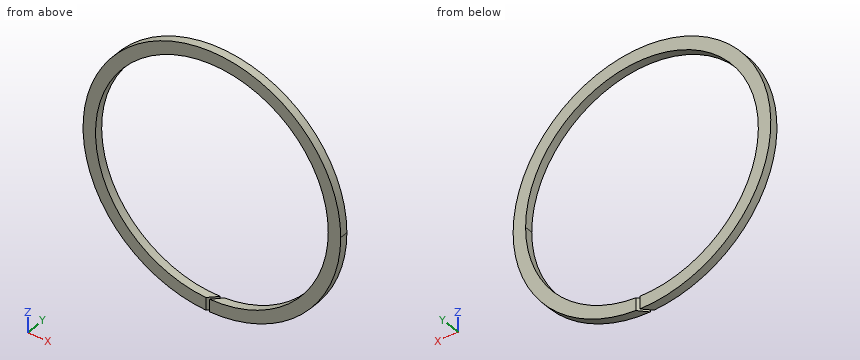
```python
from build123d import *

# Parameters (mm, degrees)
SKETCH5_R           = 46.5
SKETCH5_R_2         = 42
BOSS_EXTRUDE3_DEPTH = 1.5
CUT_EXTRUDE3_DEPTH  = 66


with BuildPart() as part:
    # Sketch5 → Boss-Extrude3 (new body, symmetric)
    with BuildSketch(Plane(origin=(0, 0, 0), x_dir=(1, 0, 0), z_dir=(0, 1, 0))):
        Circle(SKETCH5_R)
        Circle(SKETCH5_R_2, mode=Mode.SUBTRACT)
    extrude(amount=BOSS_EXTRUDE3_DEPTH, both=True)

    # Sketch6 → Cut-Extrude3 (cut)
    with BuildSketch(Plane.XY):
        Polygon((-10.568822045, -11.275928826), (11.275928826, 10.568822045), (10.568822045, 11.275928826), (-11.275928826, -10.568822045), align=None)
    extrude(amount=-CUT_EXTRUDE3_DEPTH, mode=Mode.SUBTRACT)


solid = part.part
```
Model file for the job. Use its own axes, mm. Give positions to 0.01 mm unless a question says otherwise; leave off trailing zeros. Order: outer loops, then holes, each group sorted by start corner. A loop starts at its lowest first (then second) coordinate and runs counter-clockwise, first axis right, second up.
1) Saw through at C-C, the plane y = -1. Write the cut outline in (x, z), then the cut area to 3 significant figures.
2) Saw through at A-A, the plane z = -28. Write the cut outline in (x, y).
3) Saw through at B-B, the plane x = -16.5. Write the cut outline in (y, z).
4) Wall check: probe 1 along X at (y, z) = (-0.65, 0); probe 2 along Z at (x, y) = (0, 0); probe 3 along X at (y, z) = (0.9, 26). Give the ranges that are in metal, low to high.
5) Pin check, flat tips, straight feed: pin 1 (1 mm diameter, centred on y = 1, z = 31, fed in from +X); pin 2 (1 mm diameter, centred on y = 1, z = 21, fed in from -X). Stop position of each tip, or through.
Computed:
1. outline: (-1.71, -46.47) - (-1.71, -41.97) arc R42 cw (long way) to (-0.29, -42) - (-0.29, -46.5) arc R46.5 ccw (long way) to start
1. area: 1,240 mm2
2. outline: (-37.12, -1.5) - (-31.3, -1.5) - (-31.3, 1.5) - (-37.12, 1.5) - close; (31.3, -1.5) - (37.12, -1.5) - (37.12, 1.5) - (31.3, 1.5) - close
3. outline: (-1.5, -43.47) - (1.5, -43.47) - (1.5, -38.62) - (-1.5, -38.62) - close; (-1.5, 38.62) - (1.5, 38.62) - (1.5, 43.47) - (-1.5, 43.47) - close
4. probe 1: x = -46.5 to -42, 42 to 46.5
4. probe 2: z = 42 to 46.5
4. probe 3: x = -38.55 to -32.98, 32.98 to 38.55
5. pin 1: stops at x = 35.1
5. pin 2: stops at x = -41.74
